Could you check a few things on this model? Use its own coordinates, in mm. A direction names the side the tool comes from. Coordinates: 2 decimals unless noted, no trailing zeros. Loops run counter-clockwise (first coordinate to the right, second up) from the corner with the lowest first, then second, coordinate; pieces in that order, holes last.
1) Imagine slicing it at A-A on x = -226. Please give me the cut outline in (y, z).
2) Thinking about a two-plate mould opening in Z: for faces 1 (the face through (-153, -45, 71)), 2 (the face through (-145, -1, 69)), 3 (the face through (-525, 0, 10)), which applies, released by +Z, released by -Z, zero draft, split by the parting line, or undercut?
3) For faces 4 (the face through (-71, 20, 100)), 5 (the face through (-153, -1, 130)), 6 (the face through (-81, -20, 80)), which set-ups out of +Z, -Z, +X, -X, +Y, -Y let a thin tool reach every point of the face, with its end or its side?
4) Will these pins go through, and if not, where does the flat tip stop? P1, Ø10, axis at x = -155, y = 31, coming from the -Z side; P2, Ø12, axis at x = -68, z = 21, coming from the +Y side; P3, Ø12, axis at x = -42, y = 22, coming from the +Z side; P4, Ø16.5, axis at y = -1.5, z = 3.5, coming from the +X side.
5) If I drill on line 1 along X through (y, z) = (-27, 36.5); line 2 along Z through (x, y) = (0, -18); line 3 along X through (y, z) = (19, 0), over which ranges is the centre line in solid material (lowest first)?
```python
from build123d import *

# Parameters (mm, degrees)
F0_R           = 5
F1_DEPTH       = 27.5
F1_DEPTH_BACK  = 27.5
F4_R           = 5
F5_DEPTH       = 55
F7_DEPTH       = 12.5
F7_DEPTH_BACK  = 12.5
F9_W           = 15
F9_H           = 120
F10_DEPTH      = 45
F10_DEPTH_BACK = 45
F11_R          = 5
F12_R          = 5
F14_R          = 10
F16_R          = 5
F17_R          = 0.5


with BuildPart() as f1:
    # F0 (on Front) → F1 (new body, two sides)
    with BuildSketch(Plane.XZ) as f1_sk:
        with BuildLine():
            Line((-900, -10), (0, -10))
            ThreePointArc((0, -10), (10, 0), (0, 10))
            Line((0, 10), (-900, 10))
            Line((-900, 10), (-900, -10))
        make_face()
        Circle(F0_R, mode=Mode.SUBTRACT)
    extrude(amount=-F1_DEPTH)
    extrude(f1_sk.sketch, amount=F1_DEPTH_BACK)

    # F4 (on offset) → F5 (join)
    with BuildSketch(Plane.XZ.offset(27.5)):
        with BuildLine():
            Line((-10, 80), (-10, 0))
            ThreePointArc((-10, 0), (0, -10), (10, 0))
            Line((10, 0), (10, 90))
            ThreePointArc((10, 90), (7.0710678119, 97.0710678119), (0, 100))
            Line((0, 100), (-145, 100))
            Line((-145, 100), (-145, 80))
            Line((-145, 80), (-10, 80))
        make_face()
        Circle(F4_R, mode=Mode.SUBTRACT)
    extrude(amount=-F5_DEPTH)

    # F6 (on offset) → F7 (cut, two sides)
    with BuildSketch(Plane.XZ) as f7_sk:
        Polygon((-105, -42.0839144895), (30, -42.0839144895), (30, 107.9160855105), (-145, 107.9160855105), (-145, 27.9160855105), (-105, 28.3714774996), align=None)
    extrude(amount=-F7_DEPTH, mode=Mode.SUBTRACT)
    extrude(f7_sk.sketch, amount=F7_DEPTH_BACK, mode=Mode.SUBTRACT)

    # F9 (on offset) → F10 (join, two sides)
    with BuildSketch(Plane.XZ) as f10_sk:
        with Locations((-152.5, 70)):
            Rectangle(F9_W, F9_H)
    extrude(amount=F10_DEPTH)
    extrude(f10_sk.sketch, amount=-F10_DEPTH_BACK)

    # F11
    f11_edges = [f1.edges().sort_by_distance(p)[0] for p in [
        (-152.5, -45, 130),
        (-152.5, 45, 130),
        (-152.5, -45, 10),
        (-152.5, 45, 10),
    ]]
    fillet(f11_edges, radius=F11_R)

    # F12
    f12_edges = [f1.edges().sort_by_distance(p)[0] for p in [
        (-10, -20, 80),
        (-10, 20, 80),
    ]]
    fillet(f12_edges, radius=F12_R)

    # F15: sweep along a path in F8
    with BuildLine(Plane.XZ) as f15_path:
        ThreePointArc((-150, 0), (-91.3142143513, -119.0030010437), (38.8228567654, -144.8888739434))
    # F14 (on offset) → F15 (sweep)
    with BuildSketch(Plane(origin=(0, 0, 0), x_dir=(1, 0, 0), z_dir=(0, 0, -1))):
        with Locations((-150, 0)):
            Circle(F14_R)
    sweep(path=f15_path.line)

    # F16
    f16_edges = [f1.edges().sort_by_distance(p)[0] for p in [
        (-105, 0, -10),
    ]]
    fillet(f16_edges, radius=F16_R)

    # F17
    f17_edges = [f1.edges().sort_by_distance(p)[0] for p in [
        (41.411047, 0, -154.548132),
    ]]
    fillet(f17_edges, radius=F17_R)


solid = f1.part
```
Filled in:
1. outline: (-27.5, -10) - (27.5, -10) - (27.5, 10) - (-27.5, 10) - close
2. face 1: zero draft
2. face 2: undercut
2. face 3: released by +Z
3. face 4: +Z, +X, +Y, -Y
3. face 5: +Z, +X, -X, +Y, -Y
3. face 6: +Y, -Y
4. P1: stops at z = -10
4. P2: passes through
4. P3: stops at z = 100
4. P4: stops at x = -105
5. line 1: x = -160 to -145, -10 to 10
5. line 2: z = -10 to -5, 5 to 100
5. line 3: x = -900 to -5, 5 to 10
